Work out the finished part from the listing and answer in its coordinate system (mm). Give positions to 0.01 mm unless a question says otherwise; leave off trailing zeros. Write each loop counter-clockwise with the first axis right and the second up, starting at its lowest first coordinate (ties: lowest second). Pieces come first, ordered by that corner, then holes. Notation, with made-up numbers: (-10.75, 69.5) -> (26.25, 69.5) arc R25 cw to (26.25, 83.5) -> close; hole circle Ø3 at (40.25, 37). An arc over 180 degrees is marked (long way). Write item = value, one per line. Start each with the question number.
from build123d import *

# Parameters (mm, degrees)
SKETCH1_R           = 1.5
SKETCH1_R_2         = 4
SKETCH1_R_3         = 2
BOSS_EXTRUDE1_DEPTH = 3
SKETCH2_R           = 1.5
CUT_EXTRUDE2_DEPTH  = 3
FILLET1_R           = 1
FILLET2_R           = 1.25
FILLET3_R           = 3
FILLET4_R           = 1
FILLET5_R           = 0.5
FILLET6_R           = 3


with BuildPart() as part:
    # Sketch1 → Boss-Extrude1 (new body)
    with BuildSketch(Plane(origin=(0, 0, 0), x_dir=(1, 0, 0), z_dir=(0, 1, 0))):
        with BuildLine():
            Line((23.065289305, 10.113813665), (21.67993882, -13.846169724))
            Line((21.67993882, -13.846169724), (108.324128041, -18.855879772))
            ThreePointArc((108.324128041, -18.855879772), (130.192539316, -8.10025521), (109.709478525, 5.104103618))
            Line((109.709478525, 5.104103618), (23.065289305, 10.113813665))
        make_face()
        with Locations(Location((26.914085012, -9.154397921, 0), (0, 0, 270))):
            Circle(SKETCH1_R, mode=Mode.SUBTRACT)
        with Locations(Location((27.769141375, 4.847433338, 0), (0, 0, 270))):
            Circle(SKETCH1_R, mode=Mode.SUBTRACT)
        with Locations(Location((116.215882339, -7.292134094, 0), (0, 0, 270))):
            Circle(SKETCH1_R_2, mode=Mode.SUBTRACT)
        with Locations(Location((27.341613193, -2.153482292, 0), (0, 0, 270))):
            Circle(SKETCH1_R_3, mode=Mode.SUBTRACT)
    extrude(amount=BOSS_EXTRUDE1_DEPTH)

    # Sketch2 → Cut-Extrude2 (cut)
    with BuildSketch(Plane(origin=(0, 0, 0), x_dir=(1, 0, 0), z_dir=(0, 1, 0))):
        with Locations(Location((86.765069423, -5.589307457, 0), (0, 0, 270))):
            Circle(SKETCH2_R)
        Polygon((35.169248231, 2.903114787), (34.534295925, -8.078544267), (42.636402929, -6.543662479), (43.040463487, 0.444666009), align=None)
        Polygon((48.712983182, -5.392501139), (48.943874929, -1.399170574), (56.815090185, -3.857619351), align=None)
        Polygon((37.85954525, 6.253409084), (64.924303207, -2.199837199), (65.321257747, 4.665590925), align=None)
        Polygon((36.820532386, -11.716578458), (64.679199423, -6.438968493), (64.282244884, -13.304396617), align=None)
        Polygon((69.27390809, -13.593011301), (96.735620587, -15.180829461), (69.670862629, -6.727583177), align=None)
        Polygon((97.77463345, 2.789158082), (69.915966413, -2.488451884), (70.312920953, 4.376976241), align=None)
        Polygon((81.158794022, -7.268496587), (74.785077728, -4.896632215), (81.389685769, -3.275166022), align=None)
        Polygon((100.060869911, -0.848876109), (99.425917606, -11.830535163), (91.55470235, -9.372086386), (91.958762908, -2.383757897), align=None)
        with BuildLine():
            Line((120.953295402, -11.107486957), (122.283518403, -12.600975079))
            ThreePointArc((122.283518403, -12.600975079), (122.201885843, -14.01283064), (120.790030282, -13.931198079))
            Line((120.790030282, -13.931198079), (119.459807281, -12.437709958))
            ThreePointArc((119.459807281, -12.437709958), (119.541439841, -11.025854397), (120.953295402, -11.107486957))
        make_face()
        with BuildLine():
            Line((114.170015477, -16.689709781), (114.256599882, -15.192210819))
            ThreePointArc((114.256599882, -15.192210819), (115.840683249, -13.781296262), (117.251597806, -15.36537963))
            Line((117.251597806, -15.36537963), (117.165013401, -16.862878591))
            ThreePointArc((117.165013401, -16.862878591), (115.580930034, -18.273793148), (114.170015477, -16.689709781))
        make_face()
        with BuildLine():
            Line((121.361458203, -4.048209152), (122.854946324, -2.717986152))
            ThreePointArc((122.854946324, -2.717986152), (122.936578884, -1.306130591), (121.524723323, -1.22449803))
            Line((121.524723323, -1.22449803), (120.031235202, -2.554721031))
            ThreePointArc((120.031235202, -2.554721031), (119.949602642, -3.966576592), (121.361458203, -4.048209152))
        make_face()
        with BuildLine():
            Line((115.266751277, 2.278610403), (115.180166872, 0.781111441))
            ThreePointArc((115.180166872, 0.781111441), (116.591081429, -0.802971926), (118.175164796, 0.60794263))
            Line((118.175164796, 0.60794263), (118.261749201, 2.105441592))
            ThreePointArc((118.261749201, 2.105441592), (116.850834644, 3.689524959), (115.266751277, 2.278610403))
        make_face()
        with BuildLine():
            Line((112.971957397, -2.14655823), (111.641734396, -0.653070109))
            ThreePointArc((111.641734396, -0.653070109), (110.229878835, -0.571437549), (110.148246275, -1.98329311))
            Line((110.148246275, -1.98329311), (111.478469276, -3.476781231))
            ThreePointArc((111.478469276, -3.476781231), (112.890324837, -3.558413791), (112.971957397, -2.14655823))
        make_face()
        with BuildLine():
            Line((112.400529476, -12.029547157), (110.907041355, -13.359770158))
            ThreePointArc((110.907041355, -13.359770158), (109.495185794, -13.278137598), (109.576818354, -11.866282037))
            Line((109.576818354, -11.866282037), (111.070306475, -10.536059036))
            ThreePointArc((111.070306475, -10.536059036), (112.482162036, -10.617691596), (112.400529476, -12.029547157))
        make_face()
        with BuildLine():
            Line((125.786626836, -6.343003033), (124.289127874, -6.256418627))
            ThreePointArc((124.289127874, -6.256418627), (122.705044507, -7.667333184), (124.115959064, -9.251416551))
            Line((124.115959064, -9.251416551), (125.613458025, -9.338000956))
            ThreePointArc((125.613458025, -9.338000956), (127.197541393, -7.9270864), (125.786626836, -6.343003033))
        make_face()
        with BuildLine():
            Line((106.818306653, -5.246267232), (108.315805614, -5.332851638))
            ThreePointArc((108.315805614, -5.332851638), (109.726720171, -6.916935005), (108.142636804, -8.327849561))
            Line((108.142636804, -8.327849561), (106.645137842, -8.241265156))
            ThreePointArc((106.645137842, -8.241265156), (105.234223285, -6.657181789), (106.818306653, -5.246267232))
        make_face()
        with BuildLine():
            ThreePointArc((122.434928959, -17.554855914), (124.197220344, -16.253062821), (125.693448496, -14.652551185))
            ThreePointArc((125.693448496, -14.652551185), (125.517019407, -13.249385914), (124.113854136, -13.425815003))
            ThreePointArc((124.113854136, -13.425815003), (122.866997343, -14.7595747), (121.398421189, -15.844402277))
            ThreePointArc((121.398421189, -15.844402277), (121.061448255, -17.21788298), (122.434928959, -17.554855914))
        make_face()
        with BuildLine():
            ThreePointArc((123.576299429, 2.185432062), (125.176811066, 0.689203911), (126.478604158, -1.073087475))
            ThreePointArc((126.478604158, -1.073087475), (126.141631225, -2.446568178), (124.768150522, -2.109595245))
            ThreePointArc((124.768150522, -2.109595245), (123.683322945, -0.64101909), (122.349563248, 0.605837703))
            ThreePointArc((122.349563248, 0.605837703), (122.173134159, 2.009002974), (123.576299429, 2.185432062))
        make_face()
        with BuildLine():
            ThreePointArc((106.738316182, 0.068282996), (108.234544334, 1.668794633), (109.996835719, 2.970587725))
            ThreePointArc((109.996835719, 2.970587725), (111.370316423, 2.633614792), (111.033343489, 1.260134088))
            ThreePointArc((111.033343489, 1.260134088), (109.564767335, 0.175306511), (108.317910542, -1.158453186))
            ThreePointArc((108.317910542, -1.158453186), (106.914745271, -1.334882275), (106.738316182, 0.068282996))
        make_face()
        with BuildLine():
            ThreePointArc((105.95316052, -13.511180714), (107.254953612, -15.273472099), (108.855465249, -16.769700251))
            ThreePointArc((108.855465249, -16.769700251), (110.258630519, -16.593271162), (110.08220143, -15.190105892))
            ThreePointArc((110.08220143, -15.190105892), (108.748441733, -13.943249099), (107.663614156, -12.474672944))
            ThreePointArc((107.663614156, -12.474672944), (106.290133453, -12.137700011), (105.95316052, -13.511180714))
        make_face()
    extrude(amount=CUT_EXTRUDE2_DEPTH, mode=Mode.SUBTRACT)

    # Fillet1
    fillet1_edges = [part.edges().sort_by_distance(p)[0] for p in [
        (100.060869911, 1.5, 0.848876109),
        (91.958762908, 1.5, 2.383757897),
        (91.55470235, 1.5, 9.372086386),
        (99.425917606, 1.5, 11.830535163),
        (43.040463487, 1.5, -0.444666009),
        (35.169248231, 1.5, -2.903114787),
        (34.534295925, 1.5, 8.078544267),
        (42.636402929, 1.5, 6.543662479),
    ]]
    fillet(fillet1_edges, radius=FILLET1_R)

    # Fillet2
    fillet2_edges = [part.edges().sort_by_distance(p)[0] for p in [
        (97.77463345, 1.5, -2.789158082),
        (96.735620587, 1.5, 15.180829461),
        (36.820532386, 1.5, 11.716578458),
        (37.85954525, 1.5, -6.253409084),
    ]]
    fillet(fillet2_edges, radius=FILLET2_R)

    # Fillet3
    fillet3_edges = [part.edges().sort_by_distance(p)[0] for p in [
        (70.312920953, 1.5, -4.376976241),
        (69.27390809, 1.5, 13.593011301),
        (64.282244884, 1.5, 13.304396617),
        (65.321257747, 1.5, -4.665590925),
    ]]
    fillet(fillet3_edges, radius=FILLET3_R)

    # Fillet4
    fillet4_edges = [part.edges().sort_by_distance(p)[0] for p in [
        (69.915966413, 1.5, 2.488451884),
        (69.670862629, 1.5, 6.727583177),
        (64.679199423, 1.5, 6.438968493),
        (64.924303207, 1.5, 2.199837199),
    ]]
    fillet(fillet4_edges, radius=FILLET4_R)

    # Fillet5
    fillet5_edges = [part.edges().sort_by_distance(p)[0] for p in [
        (81.158794022, 1.5, 7.268496587),
        (81.389685769, 1.5, 3.275166022),
        (74.785077728, 1.5, 4.896632215),
        (48.712983182, 1.5, 5.392501139),
        (56.815090185, 1.5, 3.857619351),
        (48.943874929, 1.5, 1.399170574),
    ]]
    fillet(fillet5_edges, radius=FILLET5_R)

    # Fillet6
    fillet6_edges = [part.edges().sort_by_distance(p)[0] for p in [
        (108.324128041, 1.5, 18.855879772),
        (21.67993882, 1.5, 13.846169724),
        (23.065289305, 1.5, -10.113813665),
        (109.709478525, 1.5, -5.104103618),
    ]]
    fillet(fillet6_edges, radius=FILLET6_R)


solid = part.part
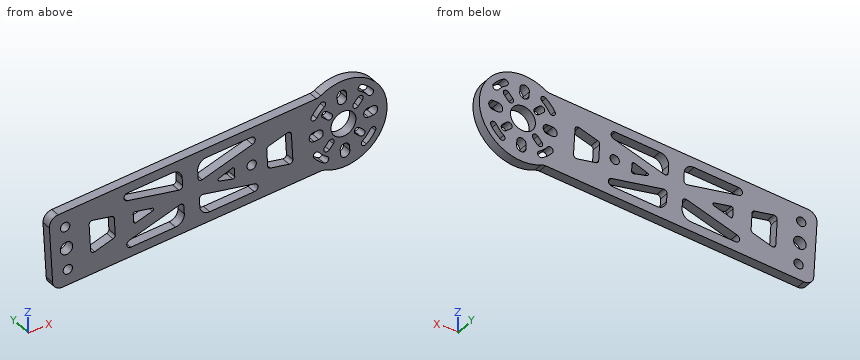
(1) A cutting plane is placed at C-C, the plane y = 0.8. State how many separate pieces and enclosed holes the cut face has, then the cut area to 3 significant figures.
(2) A cutting plane is placed at A-A, the plane x = 79. Write down the section's boundary in (y, z).
(3) A cutting plane is placed at B-B, the plane x = 95.5. Write down the section's boundary in (y, z).
(4) Find the intervals of material crossed by line 1 along Z through (x, y) = (116.5, 2.3); line 2 along X through (y, z) = (1.95, 13.5); line 3 along Z through (x, y) = (108.5, 2.05) (3 decimals), in increasing order.
Results list:
q1.separate_pieces = 1
q1.enclosed_holes = 25
q1.area = 1,880 mm²
q2.outline = (0, -6.88) -> (3, -6.88) -> (3, -3.87) -> (0, -3.87) -> close; (0, 0.77) -> (3, 0.77) -> (3, 3.86) -> (0, 3.86) -> close; (0, 6.47) -> (3, 6.47) -> (3, 9.64) -> (0, 9.64) -> close; (0, 14.16) -> (3, 14.16) -> (3, 17.16) -> (0, 17.16) -> close
q3.outline = (0, -5.93) -> (3, -5.93) -> (3, 1.71) -> (0, 1.71) -> close; (0, 10.6) -> (3, 10.6) -> (3, 18.11) -> (0, 18.11) -> close
q4.line_1 = -6.7 to -3.67, 0.79 to 3.3, 11.28 to 13.98, 18.02 to 21.29
q4.line_2 = 23.15 to 71.2, 87.91 to 105.95, 108.38 to 109.78, 110.7 to 120.41, 122.51 to 124.06, 125.75 to 128.76
q4.line_3 = -5.174 to -1.898, 0.931 to 5.355, 8.306 to 13.653, 16.483 to 19.029
